from build123d import *

# Parameters (mm, degrees)
SKETCH1_W           = 30
SKETCH1_H           = 85
BOSS_EXTRUDE1_DEPTH = 5
SKETCH2_R           = 4.5
BOSS_EXTRUDE2_DEPTH = 30
FILLET1_R           = 2


with BuildPart() as part:
    # Sketch1 → Boss-Extrude1 (new body)
    with BuildSketch(Plane(origin=(0, 0, 0), x_dir=(1, 0, 0), z_dir=(0, 1, 0))):
        Rectangle(SKETCH1_W, SKETCH1_H)
    extrude(amount=BOSS_EXTRUDE1_DEPTH)

    # Sketch2 → Boss-Extrude2 (add)
    with BuildSketch(Plane(origin=(15, 0, 0), x_dir=(0, 0, -1), z_dir=(1, 0, 0))):
        with BuildLine():
            Line((-42.5, 5), (-42.5, 8.5))
            ThreePointArc((-42.5, 8.5), (-57.01040764, 14.51040764), (-51, 0))
            Line((-51, 0), (-42.5, 0))
            Line((-42.5, 0), (-42.5, 5))
        make_face()
        with Locations((-51, 8.5)):
            Circle(SKETCH2_R, mode=Mode.SUBTRACT)
        Polygon((42.5, 5), (42.5, 0), (47.5, 0), (47.5, 30), (42.5, 30), align=None)
        Polygon((42.5, 30), (47.5, 30), (47.5, 35), (27.5, 35), (27.5, 30), align=None)
    extrude(amount=-BOSS_EXTRUDE2_DEPTH)

    # Fillet1
    fillet1_edges = [part.edges().sort_by_distance(p)[0] for p in [
        (0, 5, -42.5),
        (0, 0, -47.5),
        (0, 30, -42.5),
        (0, 30, -27.5),
        (0, 35, -27.5),
        (0, 35, -47.5),
        (0, 5, 42.5),
    ]]
    fillet(fillet1_edges, radius=FILLET1_R)


solid = part.part
The model under review builds one solid part; all positions refer to its coordinate system, in mm. A direction names the side the tool comes from. Coordinates: 2 decimals unless noted, no trailing zeros. Loops run counter-clockwise (first coordinate to the right, second up) from the corner with the lowest first, then second, coordinate; pieces in that order, holes last. Notation, with made-up numbers: (66, 1.25) -> (87, 1.25) arc R33 ccw to (87, 31.25) -> close; hole circle Ø3 at (-37.75, 11). An arc over 180 degrees is marked (long way). Use a Markdown table: item, result. Add a question column.
1. Add section C-C on y = 15.5. Write out the cut boundary in (x, z).
2. Machinability: for faces 1 (the face through (15, 4.6, -1.7)), 2 (the face through (0, 18, -42.5)), 3 (the face through (-0.21, 30.57, -28.1)), which of the approach directions +Z, -Z, +X, -X, +Y, -Y give a long, thin tool a straight path to every point of the face, cutting with its end or side? Answer none if there is none.
3. Draft analysis for pull direction Y (two halves, no side actions). For faces 4 (the face through (0.21, 5.57, -41.9)), 5 (the face through (0, 0, 3)), 6 (the face through (0.21, 5.57, 41.9)), state which applies: pulls with the +Y half, pulls with the -Y half, needs draft (parallel to the pull), parting line crosses it, or undercut.
4. Add section A-A on y = 11. Write out the cut boundary in (x, z).
5. To check wall thickness, follow line 1 (Y direction, x = 5.5, z = 51); line 2 (Z direction, x = -7.5, y = 8); line 3 (Y direction, x = 12.25, z = -35). State the ranges of each line that lie inside material, in increasing order.
6. Clearance check with flat-ended pins moving along their axes: pin 1 Ø3 at (x, y) = (-5.5, 24) entering from +Z; pin 2 Ø8 at (x, z) = (11, 44.5) entering from +Y; pin 3 Ø15 at (x, z) = (-7, -1.5) entering from +Y. State where each tip first meets the part, or that it passes through.
7. Add section B-B on x = 1.75. Write out the cut boundary in (y, z).
8. Add section D-D on z = 32. Write out the cut boundary in (x, y).
Returned:
| question | item | result |
|---|---|---|
| 1 | outline | (-15, -47.5) -> (15, -47.5) -> (15, -42.5) -> (-15, -42.5) -> close; (-15, 46.18) -> (15, 46.18) -> (15, 55.82) -> (-15, 55.82) -> close |
| 2 | face 1 | +Z, -Z, +X, +Y, -Y |
| 2 | face 2 | +X, -X |
| 2 | face 3 | +Z, +X, -X |
| 3 | face 4 | undercut |
| 3 | face 5 | pulls with the -Y half |
| 3 | face 6 | pulls with the +Y half |
| 4 | outline | (-15, -47.5) -> (15, -47.5) -> (15, -42.5) -> (-15, -42.5) -> close; (-15, 42.88) -> (15, 42.88) -> (15, 47.26) -> (-15, 47.26) -> close; (-15, 54.74) -> (15, 54.74) -> (15, 59.12) -> (-15, 59.12) -> close |
| 5 | line 1 | y = 0 to 4, 13 to 17 |
| 5 | line 2 | z = -47.5 to -42.5, 42.5 to 46.53, 55.47 to 59.49 |
| 5 | line 3 | y = 0 to 5, 30 to 35 |
| 6 | pin 1 | stops at z = -42.5 |
| 6 | pin 2 | stops at y = 16.62 |
| 6 | pin 3 | stops at y = 5 |
| 7 | outline | (0, -45.5) arc R2 ccw to (2, -47.5) -> (33, -47.5) arc R2 ccw to (35, -45.5) -> (35, -29.5) arc R2 ccw to (33, -27.5) -> (32, -27.5) arc R2 ccw to (30, -29.5) -> (30, -40.5) arc R2 cw to (28, -42.5) -> (7, -42.5) arc R2 cw to (5, -40.5) -> (5, 40.5) arc R2 cw to (7, 42.5) -> (8.5, 42.5) arc R8.5 ccw (long way) to (0, 51) -> close; hole circle Ø9 at (8.5, 51) |
| 8 | outline | (-15, 0) -> (15, 0) -> (15, 5) -> (-15, 5) -> close |
